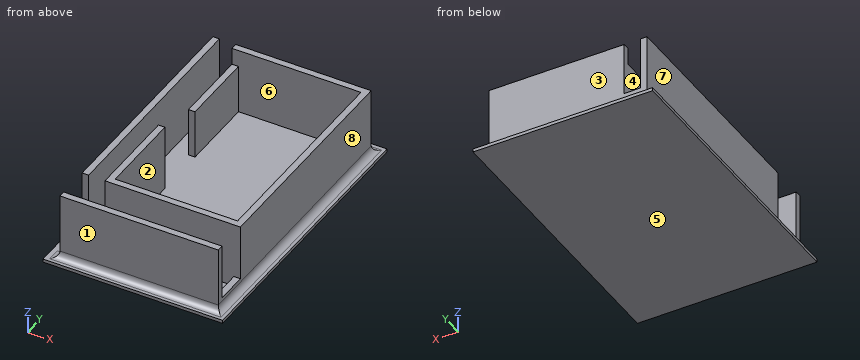
Autodesk Inventor part; units mm, degrees
ref_plane "Plano de trabajo2" through (0, 0, 1.5) normal (0, 0, 1) x (1, 0, 0)
ref_plane "YZ Plane" through (0, 0, 0) normal (1, 0, 0) x (0, 1, 0)
ref_plane "XZ Plane" through (0, 0, 0) normal (0, 1, 0) x (-1, 0, 0)
ref_plane "Plano de trabajo1" through (0, 0, 0) normal (0, 0, 1) x (1, 0, 0)
sketch "Boceto1" plane through (0, 0, 0) normal (0, 0, 1) x (1, 0, 0)
  line L0 (0.4509, -110.4895) -> (0.451, -110.4898)
  line L1 (0.4512, -110.4895) -> (0.4509, -110.4895)
  line L2 (-0.0742, -109.5793) -> (0.4512, -110.4895)
  line L3 (-0.5999, -110.4893) -> (0.1885, -110.0344)
  line L4 (0.4512, -110.4895) -> (-0.3337, -110.0363)
  line L5 (0.4512, -110.4895) -> (-0.5999, -110.4895)
  line L6 (-0.5999, -110.4895) -> (-0.0743, -109.5792)
  line L7 (-0.0743, -109.5792) -> (0.4512, -110.4895)
  line L8 (-95.0743, -55.3377) -> (94.9257, -55.3377)
  line L9 (94.9257, -55.3377) -> (-0.0743, -219.8826)
  line L10 (-0.0743, -219.8826) -> (-95.0743, -55.3377)
  point P0 (0, 0)
  point P1 (-0.0743, -110.186)
  point P2 (-0.0743, -110.186)
  point P3 (0.1885, -110.0344)
  dimension "d0" = 190
extrude "Extrusión1" add sketch "Boceto1" along normal blind 1.5 contours L2 L3 L6 | L2 L4 L3 | L3 L4 L5 | L8 L9 L10
fillet "Empalme1" radius 30 3 edges at (-95.0743, -55.3377, 0.75) (94.9257, -55.3377, 0.75) (-0.0743, -219.8826, 0.75)
sketch "Boceto2" plane through (0, 0, 1.5) normal (0, 0, 1) x (1, 0, 0)
  line L0 (25.9064, -174.8826) -> (68.9449, -100.3377)
  line L1 (42.9642, -55.3377) -> (-43.1128, -55.3377)
  line L2 (-69.0936, -100.3377) -> (-26.0551, -174.8826)
  line L3 (0.4512, -110.4895) -> (0.1885, -110.0344)
  line L4 (0.1885, -110.0344) -> (0.1885, -110.0344)
  line L5 (0.1885, -110.0344) -> (0.4512, -110.4895)
  line L6 (-0.0743, -219.8826) -> (94.9257, -55.3377)
  line L7 (-0.0743, -219.8826) -> (-0.0743, -55.3377)
  line L8 (-18.8243, -77.186) -> (18.6757, -77.186)
  line L9 (18.6757, -77.186) -> (18.6757, -143.186)
  line L10 (18.6757, -143.186) -> (-18.8243, -143.186)
  line L11 (-18.8243, -143.186) -> (-18.8243, -77.186)
  line L12 (-18.8243, -77.186) -> (18.6757, -143.186) construction
  line L13 (18.6757, -77.186) -> (-18.8243, -143.186) construction
  line L14 (-20.8243, -75.186) -> (20.6757, -75.186)
  line L15 (20.6757, -75.186) -> (20.6757, -145.186)
  line L16 (20.6757, -145.186) -> (-20.8243, -145.186)
  line L17 (-20.8243, -145.186) -> (-20.8243, -75.186)
  line L18 (94.9257, -55.3377) -> (57.0834, -77.186)
  arc A0 (-26.0551, -174.8826) -> (25.9064, -174.8826) centre (-0.0743, -159.8826) ccw
  arc A1 (68.9449, -100.3377) -> (42.9642, -55.3377) centre (42.9642, -85.3377) ccw
  arc A2 (-43.1128, -55.3377) -> (-69.0936, -100.3377) centre (-43.1128, -85.3377) ccw
  point P0 (0, 0)
  dimension "d4" = 37.5
  dimension "d5" = 66
  dimension "d6" = 2
extrude "Extrusión2" add sketch "Boceto2" along normal blind 20.25 contours L16 L17 L14 L7 L8 L11 L10 | L7 L10 L9 L8 L14 L15 L16
sketch "Boceto3" plane through (-20.8243, -145.186, 21.75) normal (-1, 0, 0) x (0, 0, 1)
  line L0 (-20.25, 0) -> (0, 0)
  line L1 (0, 70) -> (0, 0)
  line L2 (-20.25, 70) -> (0, 70)
  line L3 (0, 70) -> (-18.05, 70)
  line L4 (-18.05, 70) -> (-18.05, 44.7)
  line L5 (-18.05, 44.7) -> (0, 44.7)
  line L6 (0, 44.7) -> (0, 70)
  line L7 (-20.25, 0) -> (-20.25, 70)
  line L8 (0, 0) -> (-17, 0)
  line L9 (-17, 0) -> (-17, 28.6)
  line L10 (-17, 28.6) -> (0, 28.6)
  line L11 (0, 28.6) -> (0, 0)
  line L12 (-18.05, 44.7) -> (-20.25, 44.7)
  line L13 (-17, 28.6) -> (-20.25, 28.6)
  point P0 (-21.75, 145.186)
  point P1 (0, 28.6)
  point P2 (0, 44.7)
  dimension "d10" = 18.05
  dimension "d11" = 25.3
  dimension "d12" = 17
  dimension "d13" = 28.6
sketch "Boceto4" plane through (0, 0, 1.5) normal (0, 0, 1) x (1, 0, 0)
  line L0 (20.6757, -145.186) -> (20.6757, -75.186)
  line L1 (20.6757, -75.186) -> (-20.8243, -75.186)
  line L2 (-20.8243, -75.186) -> (-20.8243, -145.186)
  line L3 (-20.8243, -145.186) -> (20.6757, -145.186)
  line L4 (18.6757, -143.186) -> (-18.8243, -143.186)
  line L5 (-18.8243, -143.186) -> (-18.8243, -77.186)
  line L6 (-18.8243, -77.186) -> (18.6757, -77.186)
  line L7 (18.6757, -77.186) -> (18.6757, -143.186)
  line L8 (-25.8243, -75.186) -> (-25.8243, -145.186)
  line L9 (-25.8243, -75.186) -> (-27.8243, -75.186)
  line L10 (-27.8243, -75.186) -> (-27.8243, -156.986)
  line L11 (-27.8243, -145.186) -> (-25.8243, -145.186)
  line L12 (-20.8243, -154.986) -> (-20.8243, -156.986)
  line L13 (-20.8243, -156.986) -> (20.6757, -156.986)
  line L14 (20.6757, -156.986) -> (20.6757, -154.986)
  line L15 (20.6757, -154.986) -> (-20.8243, -154.986)
  line L16 (-20.8243, -156.986) -> (-27.8243, -156.986)
  line L17 (-25.8243, -145.186) -> (-25.8243, -154.986)
  line L18 (-25.8243, -154.986) -> (-20.8243, -154.986)
  line L19 (20.6757, -145.186) -> (20.6757, -154.986)
  line L20 (20.6757, -145.186) -> (18.6757, -145.186)
  line L21 (18.6757, -145.186) -> (18.6757, -154.986)
  line L22 (-20.8243, -75.186) -> (-25.8243, -75.186)
  line L23 (-20.8243, -75.186) -> (-20.8243, -77.186)
  line L24 (-20.8243, -77.186) -> (-25.8243, -77.186)
  point P0 (0, 0)
  dimension "d19" = 2
  dimension "d22" = 2
  dimension "d23" = 2
extrude "Extrusión3" add sketch "Boceto4" along normal blind 20.25 contours L19 L15 L21 L3 | L14 L13 L12 L15 | L2 L24 L8 L22 | L8 L11 L10 L9 | L12 L16 L10 L11 L17 L18
extrude "Extrusión4" cut sketch "Boceto3" against normal up to surface (2 mm away) contours L7 L12 L5 L1 L10 L13
sketch "Boceto5" plane through (-20.8243, -77.186, 1.5) normal (-1, 0, 0) x (0, 0, 1)
  line L0 (0, 0) -> (15, 0)
  line L1 (15, 0) -> (15, -23.3)
  line L2 (15, -23.3) -> (0, -23.3)
  line L3 (0, -23.3) -> (0, 0)
  line L4 (0, -23.3) -> (20.25, -23.3)
  line L5 (20.25, 0) -> (20.25, -23.3)
  line L6 (20.25, 0) -> (0, 0)
  line L7 (0, -23.3) -> (0, 0)
  point P0 (-1.5, 77.186)
  point P1 (15, -23.3)
  dimension "d26" = 15
  dimension "d27" = 23.3
extrude "Extrusión5" cut sketch "Boceto5" against normal up to surface (2 mm away) contours L6 L5 L4 L1
sketch "Boceto6" plane through (-25.8243, -154.986, 1.5) normal (1, 0, 0) x (0, 0, -1)
  line L0 (0, 9.8) -> (-20.25, 9.8)
  line L1 (0, 77.8) -> (0, 0)
  line L2 (0, 77.8) -> (-20.25, 77.8)
  line L3 (-20.25, 0) -> (-20.25, 77.8)
  line L4 (0, 0) -> (-20.25, 0)
  line L5 (0, 0) -> (-11.6, 0)
  line L6 (-11.6, 0) -> (-11.6, 9.8)
  line L7 (-11.6, 9.8) -> (0, 9.8)
  line L8 (0, 9.8) -> (0, 0)
  point P0 (1.5, 154.986)
  dimension "d30" = 11.6
extrude "Extrusión6" cut sketch "Boceto6" against normal up to surface (2 mm away) contours L1 L4 L6 L0 | L6 L4 L3 L0
sketch "Boceto7" plane through (-18.8243, -77.186, 1.5) normal (0, -1, 0) x (1, 0, 0)
  line L0 (-2, 0) -> (-7, 0)
  line L1 (-2, 15) -> (-2, 0)
  line L2 (-2, 15) -> (0, 15)
  line L3 (0, 0) -> (0, 15)
  line L4 (37.5, 0) -> (0, 0)
  line L5 (37.5, 0) -> (37.5, 20.25)
  line L6 (-7, 20.25) -> (37.5, 20.25)
  line L7 (-7, 0) -> (-7, 20.25)
  line L8 (-2, 15) -> (-2, 20.25)
  line L9 (-7, 0) -> (-2, 0)
  line L10 (-2, 0) -> (-2, 4)
  line L11 (-2, 4) -> (-7, 4)
  line L12 (-7, 4) -> (-7, 0)
  point P0 (18.8243, -1.5)
  point P1 (-7, 4)
  dimension "d35" = 4
extrude "Extrusión7" cut sketch "Boceto7" against normal up to surface (2 mm away) contours L11 L7 L6 L8 L1
ref_plane "Plano de trabajo2" through (0, 0, 1.5) normal (0, 0, 1) x (1, 0, 0)
split "Dividir1" plane through (0, 0, 1.5) removes the side toward (0, 0, -1)
sketch "Boceto8" plane through (20.6757, -156.986, 1.5) normal (0, 0, -1) x (-1, 0, 0)
  line L0 (48.5, 0) -> (0, 0)
  line L1 (24.2796, 40.9499) -> (48.5, 0)
  line L2 (48.5, 81.8) -> (48.5, 11.8)
  line L3 (0, 0) -> (0, 81.8)
  line L4 (24.2796, 40.9499) -> (0, 0)
  point P0 (20.6757, 156.986)
ref_plane "Plano de trabajo3" through (-3.5743, -110.9343, 1.5) normal (0, 0, 1) x (1, 0, 0)
sketch "Boceto9" plane through (20.6757, -156.986, 21.75) normal (1, 0, 0) x (0, 0, -1)
  line L0 (20.25, 81.8) -> (20.25, 0)
  line L1 (20.25, 81.8) -> (0, 81.8)
  line L2 (0, 0) -> (0, 81.8)
  line L3 (20.25, 0) -> (0, 0)
  line L4 (20.25, 2) -> (20.25, 11.8)
  line L5 (20.25, 2) -> (0, 2)
  line L6 (0, 11.8) -> (0, 2)
  line L7 (20.25, 11.8) -> (0, 11.8)
  line L8 (0, 2) -> (20.25, 11.8)
  line L9 (17.125, 2.15) -> (3.125, 2.15)
  line L10 (3.125, 2.15) -> (3.125, 11.65)
  line L11 (3.125, 11.65) -> (17.125, 11.65)
  line L12 (17.125, 11.65) -> (17.125, 2.15)
  line L13 (17.125, 2.15) -> (3.125, 11.65) construction
  line L14 (3.125, 2.15) -> (17.125, 11.65) construction
  line L15 (3.125, 2) -> (17.125, 2)
  line L16 (17.125, 2) -> (17.125, 11.8)
  line L17 (17.125, 11.8) -> (3.125, 11.8)
  line L18 (3.125, 11.8) -> (3.125, 2)
  point P0 (21.75, 156.986)
  point P1 (12.7514, 35.7395)
  point P2 (10.125, 6.9)
  point P3 (3.125, 11.65)
  point P4 (3.125, 2.15)
  point P5 (3.125, 11.65)
  point P6 (3.125, 2.15)
  point P7 (17.125, 2.15)
  point P8 (17.125, 10.2877)
  point P9 (17.125, 11.65)
  dimension "d43" = 14
  dimension "d44" = 9.5
extrude "Extrusión8" cut sketch "Boceto9" against normal up to surface (2 mm away) contours L16 L11 L18 L7 | L12 L9 L10 L8 | L8 L10 L11 L12 | L7 L18 L10 L8 L2 | L5 L18 L9 L16 | L10 L18 L5 L8
sketch "Boceto10" plane through (20.6757, -156.986, 1.5) normal (0, 0, -1) x (-1, 0, 0)
  line L0 (49, 82) -> (0, 82)
  line L1 (0, 82) -> (0, 0)
  line L2 (0, 0) -> (49, 0)
  line L3 (49, 0) -> (49, 82)
  line L4 (52, 85) -> (-3, 85)
  line L5 (-3, 85) -> (-3, -3)
  line L6 (-3, -3) -> (52, -3)
  line L7 (52, -3) -> (52, 85)
  point P0 (20.6757, 156.986)
  dimension "d47" = 3
extrude "Extrusión9" add sketch "Boceto10" along normal blind 1 contours L3 L2 L1 L0 | L7 L6 L5 L4
fillet "Empalme3" radius 2 5 edges at (-27.8243, -110.186, 1.5) (-27.8243, -155.986, 1.5) (-3.5743, -156.986, 1.5) (20.6757, -116.086, 1.5) (-3.5743, -75.186, 1.5)
properties part number "Base4Baterias"
Design review of the part built by this model. Coordinates are the model's own, in mm. Face numbers are marked on the shaded views. A direction names the side the tool comes from. Coordinates: 2 decimals unless noted, no trailing zeros. Order: outer loops, then holes, each group sorted by start corner. A loop starts at its lowest first (then second) coordinate and runs counter-clockwise, first axis right, second up. Notation, with made-up numbers: (50.5, 10.5) -> (80.5, 10.5) arc R31 cw to (80.5, 42.5) -> close; hole circle Ø3 at (37.25, 9.25). An arc over 180 degrees is marked (long way). One line per item, written item: value.
1) We need section C-C, the plane x = -5.5. Give the boundary of the cut face in (y, z), then the cut area to 3 significant figures.
Output values:
outline: (-159.99, 0.5) -> (-71.99, 0.5) -> (-71.99, 1.5) -> (-73.19, 1.5) arc R2 cw to (-75.19, 3.5) -> (-75.19, 21.75) -> (-77.19, 21.75) -> (-77.19, 1.5) -> (-143.19, 1.5) -> (-143.19, 21.75) -> (-145.19, 21.75) -> (-145.19, 1.5) -> (-154.99, 1.5) -> (-154.99, 21.75) -> (-156.99, 21.75) -> (-156.99, 3.5) arc R2 cw to (-158.99, 1.5) -> (-159.99, 1.5) -> close
area: 211 mm2
2) We need section B-B, the plane y = -97. Give the boundary of the cut face in (x, z), then the cut area to 3 significant figures.
Output values:
outline: (-31.32, 0.5) -> (23.68, 0.5) -> (23.68, 1.5) -> (22.68, 1.5) arc R2 cw to (20.68, 3.5) -> (20.68, 21.75) -> (18.68, 21.75) -> (18.68, 1.5) -> (-18.82, 1.5) -> (-18.82, 16.5) -> (-20.82, 16.5) -> (-20.82, 1.5) -> (-25.82, 1.5) -> (-25.82, 21.75) -> (-27.82, 21.75) -> (-27.82, 3.5) arc R2 cw to (-29.82, 1.5) -> (-31.32, 1.5) -> close
area: 168 mm2
3) Draft analysis for pull direction Y (two halves, no side actions). For the marked faces 1, 2, 3 and 4, state which applies: +Y half, -Y half, draft (parallel to the pull), parting line (faces both ways), or undercut.
Output values:
face 1: -Y half
face 2: undercut
face 3: +Y half
face 4: undercut
4) We need section A-A, the plane z = 19. Give the boundary of the cut face in (x, y), then the cut area to 3 significant figures.
Output values:
outline: (-27.82, -156.99) -> (20.68, -156.99) -> (20.68, -154.99) -> (-27.82, -154.99) -> close; (-27.82, -145.19) -> (-25.82, -145.19) -> (-25.82, -75.19) -> (-27.82, -75.19) -> close; (-20.82, -145.19) -> (20.68, -145.19) -> (20.68, -75.19) -> (-20.82, -75.19) -> (-20.82, -77.19) -> (18.68, -77.19) -> (18.68, -143.19) -> (-18.82, -143.19) -> (-18.82, -116.59) -> (-20.82, -116.59) -> close
area: 588 mm2
5) Clearance check with flat-ended pins moving along their axes: P1, Ø2, axis at x = 6.5, z = 3, coming from the -Y side; P2, Ø6, axis at x = -4, z = 13.5, coming from the -Y side; P3, Ø6, axis at y = -118, z = 13, coming from the +X side; P4, Ø1.2, axis at x = -28.5, z = 14, coming from the -Y side. State where each tip first meets the part, or that it passes through.
Output values:
P1: stops at y = -157.66
P2: stops at y = -156.99
P3: stops at x = 20.68
P4: passes through
6) We need section D-D, the plane z = 12.75. Give the boundary of the cut face in (x, y), then the cut area to 3 significant figures.
Output values:
outline: (-27.82, -156.99) -> (20.68, -156.99) -> (20.68, -154.99) -> (-27.82, -154.99) -> close; (-27.82, -145.19) -> (-25.82, -145.19) -> (-25.82, -75.19) -> (-27.82, -75.19) -> close; (-20.82, -145.19) -> (20.68, -145.19) -> (20.68, -75.19) -> (-20.82, -75.19) -> (-20.82, -100.49) -> (-18.82, -100.49) -> (-18.82, -77.19) -> (18.68, -77.19) -> (18.68, -143.19) -> (-18.82, -143.19) -> (-18.82, -116.59) -> (-20.82, -116.59) -> close
area: 635 mm2
7) Machinability: for the marked faces 5, 6, 7 and 8, which of the approach directions +Z, -Z, +X, -X, +Y, -Y give a long, thin tool a straight path to every point of the face, cutting with its end or side? Answer none if there is none.
Output values:
face 5: -Z, +X, -X, +Y, -Y
face 6: +Z
face 7: +Z, -X, +Y, -Y
face 8: +Z, +X, +Y, -Y
8) To check wall thickness, follow probe 1 along X at (y, z) = (-122, 5); probe 2 along Y at (x, z) = (1.5, 8.5); probe 3 along Y at (x, z) = (-19, 18.75). State the ranges of each line that lie inside material, in increasing order. Write a range as [from, to].
Output values:
probe 1: x = [-27.82, -25.82], [-20.82, -18.82], [18.68, 20.68]
probe 2: y = [-156.99, -154.99], [-145.19, -143.19], [-77.19, -75.19]
probe 3: y = [-156.99, -154.99], [-145.19, -116.59], [-77.19, -75.19]
